Read the model definition and answer for the solid it produces. Units are mm, in the model's axes. Coordinates: 2 decimals unless noted, no trailing zeros. Write each loop counter-clockwise with the first axis right and the second up, starting at its lowest first coordinate (ties: lowest second). Pieces come first, ordered by that corner, then holes. Notation, with made-up numbers: (36.5, 67) -> (85.5, 67) arc R22 cw to (85.5, 78) -> close; hole circle Ø1 at (-26.75, 20.25). An arc over 180 degrees is marked (long way). One line per item, written item: value. Start each with the question number.
1. Find section B-B, the plane y = 195. Write down the section's boundary in (x, z).
2. Given P1, Ø5.5, axis at x = -272.95, y = 73.14, coming from the -Z side; P2, Ø1.5, axis at x = -293, z = 4.5, coming from the -Y side; P3, Ø3, axis at x = -317, z = 2, coming from the +Y side; P4, Ø1.5, axis at x = -208.5, z = 4, coming from the -Y side, each flat-ended and moving along its own axis, determine where each tip first touches the part or whether it passes through.
3. Consider line 1 along Y through (x, z) = (-182.5, 2); line 2 along X through (y, z) = (67.5, 5); line 3 along Y through (x, z) = (-317, 4.5). Determine where each line is inside the solid, lowest interval first.
4. Find section C-C, the plane x = -195. Write down the section's boundary in (y, z), and give its area (3 significant figures).
5. Find section A-A, the plane z = 2. State how many separate pieces and enclosed holes the cut face has, and give its area (3 significant figures).
6. For a pull along Y with two mould halves and no side action, classify faces 1 (the cylindrical face through (-184.794, 247.64, 3.131)), 2 (the flat face through (-256, 149, 0)), 3 (the cylindrical face through (-268.404, 71.705, 3.131)) as pulls with the +Y half, pulls with the -Y half, needs draft (parallel to the pull), parting line crosses it, or undercut.
Autodesk Inventor part; units mm, degrees
ref_plane "YZ Plane" through (0, 0, 0) normal (1, 0, 0) x (0, 1, 0)
ref_plane "XZ Plane" through (0, 0, 0) normal (0, 1, 0) x (-1, 0, 0)
ref_plane "XY Plane" through (0, 0, 0) normal (0, 0, 1) x (1, 0, 0)
sketch "Sketch1" plane through (0, 0, 0) normal (0, 0, 1) x (1, 0, 0)
  arc A0 (-215.5261, 215.5261) -> (-294.4142, 78.888) centre (0, 0) ccw construction
  arc A1 (-246.957, 246.957) -> (-337.3496, 90.3926) centre (0, 0) ccw
  arc A2 (-184.0953, 184.0953) -> (-251.4788, 67.3835) centre (0, 0) ccw
  arc A3 (-184.0953, 184.0953) -> (-246.957, 246.957) centre (-215.5261, 215.5261) ccw
  arc A4 (-337.3496, 90.3926) -> (-251.4788, 67.3835) centre (-294.4142, 78.888) ccw
  line L0 (0, 0) -> (-294.4142, 78.888) construction
  line L1 (0, 0) -> (294.4142, -78.888) construction
  line L2 (0, 0) -> (-215.5261, 215.5261) construction
  line L3 (0, 0) -> (-111.7396, 0) construction
  line L4 (-246.957, 246.957) -> (-184.0953, 184.0953) construction
  line L5 (-294.4142, 78.888) -> (-251.4788, 67.3835) construction
  line L6 (-337.3496, 90.3926) -> (-294.4142, 78.888) construction
  line L7 (-246.957, 246.957) -> (-215.5261, 215.5261) construction
  line L8 (-184.0953, 184.0953) -> (-215.5261, 215.5261) construction
  arc A5 (-199.8107, 199.8107) -> (-272.9465, 73.1358) centre (0, 0) ccw construction
  arc A6 (-204.3008, 204.3008) -> (-279.0801, 74.7793) centre (0, 0) ccw construction
  arc A7 (-195.3206, 195.3206) -> (-266.8129, 71.4923) centre (0, 0) ccw construction
  arc A8 (-195.3206, 195.3206) -> (-204.3008, 204.3008) centre (-199.8107, 199.8107) ccw construction
  arc A9 (-279.0801, 74.7793) -> (-266.8129, 71.4923) centre (-272.9465, 73.1358) ccw construction
  arc A10 (-231.2416, 231.2416) -> (-315.8819, 84.6403) centre (0, 0) ccw construction
  arc A11 (-235.7317, 235.7317) -> (-322.0155, 86.2838) centre (0, 0) ccw construction
  arc A12 (-226.7515, 226.7515) -> (-309.7483, 82.9968) centre (0, 0) ccw construction
  arc A13 (-226.7515, 226.7515) -> (-235.7317, 235.7317) centre (-231.2416, 231.2416) ccw construction
  arc A14 (-322.0155, 86.2838) -> (-309.7483, 82.9968) centre (-315.8819, 84.6403) ccw construction
  circle A15 centre (-320.9013, 62.9895) radius 3.175
  circle A16 centre (-277.8501, 51.4585) radius 3.175
  circle A17 centre (0, 0) radius 282.575 construction
  circle A18 centre (0, 0) radius 327.025 construction
  circle A19 centre (-183.4894, 214.896) radius 3.175
  circle A20 centre (-215.0012, 246.4139) radius 3.175
  circle A21 centre (-315.8819, 84.6403) radius 4.7625
  circle A22 centre (-272.9465, 73.1358) radius 4.7625
  dimension "d30" = 304.8
  dimension "d31" = 180
  dimension "d32" = 30
  dimension "d33" = 88.9
  dimension "d34" = 45
  dimension "d43" = 12.7
  dimension "d44" = 12.7
  dimension "d45" = 6.35
  dimension "d46" = 6.35
  dimension "d47" = 22.225
  dimension "d48" = 22.225
  dimension "d51" = 6.35
  dimension "d52" = 6.35
  dimension "d53" = 22.225
  dimension "d54" = 22.225
  dimension "d57" = 9.525
  dimension "d58" = 9.525
extrude "Extrusion1" add sketch "Sketch1" along normal blind 6.35
sketch "Sketch2" plane through (0, 0, 6.35) normal (0, 0, 1) x (1, 0, 0)
  circle A0 centre (0, 0) radius 348.5762
properties part number "TurretHoodPanel2"
Answer block:
1. outline: (-289.74, 0) -> (-176.1, 0) -> (-176.1, 6.35) -> (-289.74, 6.35) -> close
2. P1: passes through
2. P2: stops at y = 34.44
2. P3: stops at y = 149.78
2. P4: stops at y = 154.91
3. line 1: y = 185.78 to 211.88, 217.91 to 245.28
3. line 2: x = -337.38 to -251.45
3. line 3: y = 40.6 to 80.01, 89.27 to 146.58
4. outline: (172.5, 0) -> (254.95, 0) -> (254.95, 6.35) -> (172.5, 6.35) -> close
4. area: 524 mm2
5. separate pieces: 1
5. enclosed holes: 6
5. area: 20,100 mm2
6. face 1: parting line crosses it
6. face 2: needs draft
6. face 3: undercut
